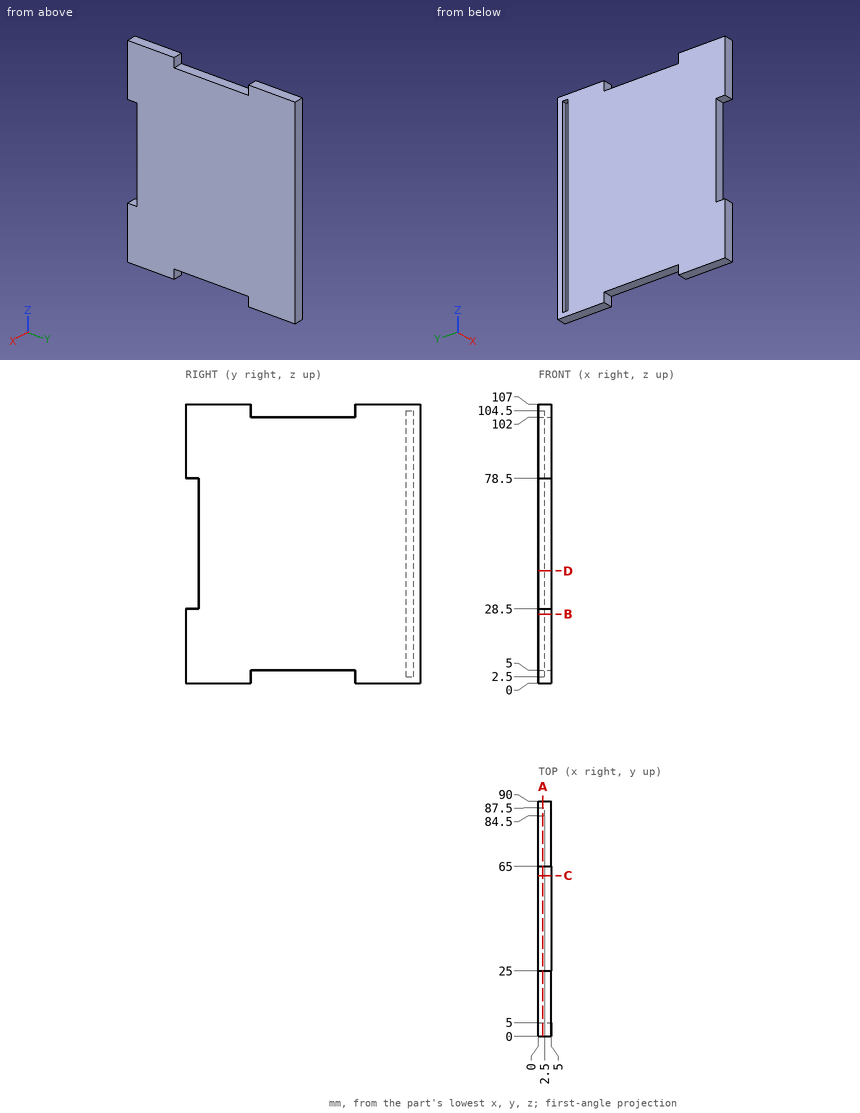
Print and shaded views of the part. All mm, measured from the part's lowest x, y and z. Give positions to 0.01 mm unless a question says otherwise; leave off trailing zeros. Order: outer loops, then holes, each group sorted by start corner. A loop starts at its lowest first (then second) coordinate and runs counter-clockwise, first axis right, second up. Notation, with made-up numbers: (31, 18) - (66, 18) arc R26 cw to (66, 44) - close; hole circle Ø8 at (66.25, -5.5). An arc over 180 degrees is marked (long way). Use a Markdown table: item, result.
1) Saw through at B-B on z = 26.5. List the corners of the cut face in (x, y).
Checked values:
| item | result |
|---|---|
| outline | (0, 0) - (5, 0) - (5, 90) - (0, 90) - (0, 87.5) - (2.5, 87.5) - (2.5, 84.5) - (0, 84.5) - close |
2) Saw through at D-D on z = 43. List the corners of the cut face in (x, y), plus the area to 4 significant figures.
Checked values:
| item | result |
|---|---|
| outline | (0, 5) - (5, 5) - (5, 90) - (0, 90) - (0, 87.5) - (2.5, 87.5) - (2.5, 84.5) - (0, 84.5) - close |
| area | 417.5 mm² |
3) Saw through at A-A on x = 1.7. List the corners of the cut face in (y, z), plus the area to 3 significant figures.
Checked values:
| item | result |
|---|---|
| outline | (0, 0) - (25, 0) - (25, 5) - (65, 5) - (65, 0) - (90, 0) - (90, 107) - (65, 107) - (65, 102) - (25, 102) - (25, 107) - (0, 107) - (0, 78.5) - (5, 78.5) - (5, 28.5) - (0, 28.5) - close; hole (84.5, 2.5) - (87.5, 2.5) - (87.5, 104.5) - (84.5, 104.5) - close |
| area | 8,670 mm² |
4) Saw through at C-C on y = 61.5. List the corners of the cut face in (x, z).
Checked values:
| item | result |
|---|---|
| outline | (0, 5) - (5, 5) - (5, 102) - (0, 102) - close |
5) Probe L1, parallel to Y at x = 1, z = 60; L2, parallel to Z at x = 1.3, y = 4.5; L3, parallel to Y at x = 2.3, z = 81. List the from-to ranges inside material, lowest first. Write a range as from..to.
Checked values:
| item | result |
|---|---|
| L1 | 5..84.5, 87.5..90 |
| L2 | 0..28.5, 78.5..107 |
| L3 | 0..84.5, 87.5..90 |
6) Flat gauge pins, fed straight in: P1, Ø2, axis at x = 1, z = 72.5, coming from the -Y side; P2, Ø0.9, axis at y = 86.5, z = 75.5, coming from the -X side; P3, Ø2.5, axis at x = 2.5, y = 39, coming from the +Z side. Where does each tip first touch, or does it go through?
Checked values:
| item | result |
|---|---|
| P1 | y = 5 |
| P2 | x = 2.5 |
| P3 | z = 102 |
